Could you check a few things on this model? Use its own coordinates, in mm. A direction names the side the tool comes from. Coordinates: 2 decimals unless noted, no trailing zeros. Loops run counter-clockwise (first coordinate to the right, second up) from the corner with the lowest first, then second, coordinate; pieces in that order, holes last. Notation, with made-up numbers: (-10, 31.25) - (22, 31.25) arc R19 ccw to (22, 46.25) - close; hole circle Ø6 at (86, 6.25). An arc over 180 degrees is marked (long way). One line per question, with ' | ' between items. Start each with the question number.
1. I want a section at A-A, the plane x = 0. Write out the boundary of the cut face in (y, z).
2. I want a section at C-C, the plane z = 33.5. Write out the boundary of the cut face in (x, y), then the cut area to 3 significant figures.
3. I want a section at D-D, the plane z = 49.5. Write out the boundary of the cut face in (x, y).
4. I want a section at B-B, the plane y = -1.5. Write out the boundary of the cut face in (x, z).
5. Please list where these lines run through material, in increasing order: L1, parallel to Y at x = 5, z = 8; L2, parallel to X at y = -0.5, z = 6; L3, parallel to Z at x = 3.25, y = -2.25. Write a range as [from, to].
6. I'm going to push flat-ended pins straight in: P1, Ø1.4, axis at y = 1, z = 3.5, coming from the +X side; P2, Ø3.5, axis at x = 1, z = 4.5, coming from the +Y side; P3, Ø2.5, axis at y = -1.5, z = 40.5, coming from the +X side. Where does each tip first touch, or does it pass through?
7. We'd pull the mould along Y, two halves only. Please class faces 6 (the flat face through (0, 0, 57)), 7 (the flat face through (-5.75, -1, 5)), 8 (the flat face through (0, 4, 27)): pulls with the +Y half, pulls with the -Y half, needs draft (parallel to the pull), parting line crosses it, or undercut.
8. Which directions (+Z, -Z, +X, -X, +Y, -Y) give clear straight access to the entire face, cutting with the end or side of a thin tool? Please do faces 1 (the flat face through (-4, 1, 43)), 2 (the flat face through (6.05, 0, 6)), 3 (the flat face through (5.75, -1, 5)), 4 (the flat face through (0, 2.3, 6)), 5 (the flat face through (0, -2.3, 6)).
from build123d import *

# Parameters (mm, degrees)
ESQUISSE1_W             = 12.1
ESQUISSE1_H             = 4.6
BOSS_EXTRU_1_DEPTH      = 12
ESQUISSE3_W             = 11.5
ESQUISSE3_H             = 2.3
ENL_V_MAT_EXTRU_1_DEPTH = 9.6
ESQUISSE2_W             = 16
ESQUISSE2_H             = 8
BOSS_EXTRU_2_DEPTH      = 31
ENL_V_MAT_EXTRU_2_DEPTH = 45.463468151
ESQUISSE5_R             = 3.6
BOSS_EXTRU_3_DEPTH      = 8
ESQUISSE6_R             = 2.55
BOSS_EXTRU_4_DEPTH      = 6


with BuildPart() as part:
    # Esquisse1 → Boss.-Extru.1 (new body)
    with BuildSketch(Plane.XY):
        Rectangle(ESQUISSE1_W, ESQUISSE1_H)
    extrude(amount=BOSS_EXTRU_1_DEPTH)

    # Esquisse3 → Enlèv. mat.-Extru.1 (cut)
    with BuildSketch(Plane(origin=(0, 0, 0), x_dir=(-1, 0, 0), z_dir=(0, 0, -1))):
        with Locations((0, -0.85)):
            Rectangle(ESQUISSE3_W, ESQUISSE3_H)
    extrude(amount=-ENL_V_MAT_EXTRU_1_DEPTH, mode=Mode.SUBTRACT)

    # Esquisse2 → Boss.-Extru.2 (add)
    with BuildSketch(Plane.XY.offset(12)):
        Rectangle(ESQUISSE2_W, ESQUISSE2_H)
    extrude(amount=BOSS_EXTRU_2_DEPTH)

    # Esquisse4 → Enlèv. mat.-Extru.2 (cut, through all)
    with BuildSketch(Plane(origin=(0, 4, 0), x_dir=(1, 0, 0), z_dir=(0, 1, 0))):
        Polygon((-8, -43), (-8, -32), (-5.2, -35), (-5.2, -43), align=None)
        Polygon((5.2, -43), (8, -43), (8, -32), (5.2, -35), align=None)
    extrude(amount=-ENL_V_MAT_EXTRU_2_DEPTH, mode=Mode.SUBTRACT)

    # Esquisse5 → Boss.-Extru.3 (add)
    with BuildSketch(Plane.XY.offset(43)):
        Circle(ESQUISSE5_R)
    extrude(amount=BOSS_EXTRU_3_DEPTH)

    # Esquisse6 → Boss.-Extru.4 (add)
    with BuildSketch(Plane.XY.offset(51)):
        Circle(ESQUISSE6_R)
    extrude(amount=BOSS_EXTRU_4_DEPTH)


solid = part.part
Results are:
1) outline: (-4, 12) - (-2.3, 12) - (-2.3, 0) - (-2, 0) - (-2, 9.6) - (0.3, 9.6) - (0.3, 0) - (2.3, 0) - (2.3, 12) - (4, 12) - (4, 43) - (3.6, 43) - (3.6, 51) - (2.55, 51) - (2.55, 57) - (-2.55, 57) - (-2.55, 51) - (-3.6, 51) - (-3.6, 43) - (-4, 43) - close
2) outline: (-6.6, -4) - (6.6, -4) - (6.6, 4) - (-6.6, 4) - close | area: 106 mm2
3) outline: circle Ø7.2 at (0, 0)
4) outline: (-8, 12) - (-6.05, 12) - (-6.05, 0) - (-5.75, 0) - (-5.75, 9.6) - (5.75, 9.6) - (5.75, 0) - (6.05, 0) - (6.05, 12) - (8, 12) - (8, 32) - (5.2, 35) - (5.2, 43) - (3.27, 43) - (3.27, 51) - (2.06, 51) - (2.06, 57) - (-2.06, 57) - (-2.06, 51) - (-3.27, 51) - (-3.27, 43) - (-5.2, 43) - (-5.2, 35) - (-8, 32) - close
5) L1: y = [-2.3, -2], [0.3, 2.3] | L2: x = [-6.05, -5.75], [5.75, 6.05] | L3: z = [0, 43]
6) P1: stops at x = 6.05 | P2: stops at y = 2.3 | P3: stops at x = 5.2
7) face 6: needs draft | face 7: undercut | face 8: pulls with the +Y half
8) face 1: +Z | face 2: -Z, +X, +Y, -Y | face 3: -Z | face 4: -Z, +X, -X, +Y | face 5: -Z, +X, -X, -Y
